Autodesk Inventor part; units mm, degrees
ref_plane "YZ Plane" through (0, 0, 0) normal (1, 0, 0) x (0, 1, 0)
ref_plane "XZ Plane" through (0, 0, 0) normal (0, 1, 0) x (-1, 0, 0)
ref_plane "XY Plane" through (0, 0, 0) normal (0, 0, 1) x (1, 0, 0)
sketch "Sketch1" plane through (0, 0, 0) normal (0, 0, 1) x (1, 0, 0)
  line L0 (0, 0) -> (-186, 0)
  line L1 (-186, 0) -> (-186, 30)
  line L2 (-186, 30) -> (0, 30)
  line L3 (0, 30) -> (0, 0)
  dimension "d0" = 186
  dimension "d1" = 30
extrude "Extrusion1" add sketch "Sketch1" along normal blind 3
sketch "Sketch2" plane through (0, 0, 0) normal (0, 0, -1) x (-1, 0, 0)
  line L0 (0, 0) -> (186, 0)
  line L1 (0, 0) -> (33, 0)
  line L2 (33, 0) -> (33, 13)
  line L3 (33, 13) -> (0, 13)
  line L4 (0, 13) -> (0, 0)
  line L5 (0, 30) -> (186, 30)
  line L6 (0, 30) -> (32.9946, 30)
  line L7 (32.9946, 30) -> (32.9946, 23)
  line L8 (32.9946, 23) -> (0, 23)
  line L9 (0, 23) -> (0, 30)
  line L10 (186, 0) -> (153, 0)
  line L11 (153, 0) -> (153, 13)
  line L12 (153, 13) -> (186, 13)
  line L13 (186, 13) -> (186, 0)
  line L14 (186, 30) -> (153, 30)
  line L15 (153, 30) -> (153, 23)
  line L16 (153, 23) -> (186, 23)
  line L17 (186, 23) -> (186, 30)
  dimension "d16" = 33
  dimension "d17" = 13
  dimension "d18" = 32.9946
  dimension "d19" = 7
  dimension "d20" = 33
hole "Hole1" at (-32.9946, 23, 0) at (-33, 13, 0) at (-153, 23, 0) at (-153, 13, 0) direction (0, 0, 1) diameter 3.4 end through all countersink diameter 6.9 countersink angle 89.954
properties part number "tyl"
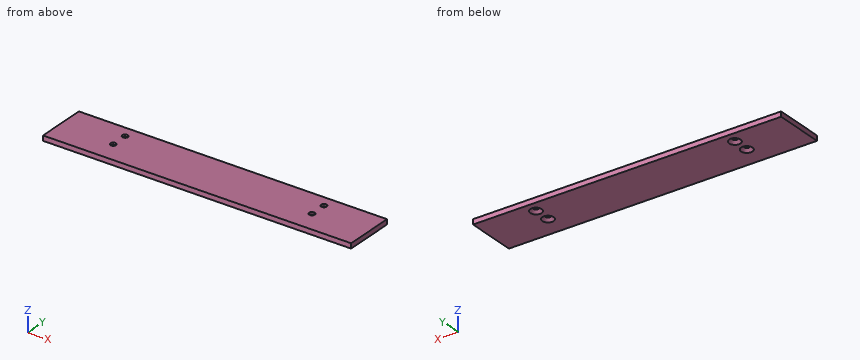
Build history of the part. All positions in model axes, mm. Coordinates: 2 decimals unless noted, no trailing zeros. Order: outer loops, then holes, each group sorted by start corner. A loop starts at its lowest first (then second) coordinate and runs counter-clockwise, first axis right, second up. Notation, with made-up numbers: (-28.5, -32) - (12.5, -32) arc R13 ccw to (12.5, -12) - close; hole circle Ø6 at (39, 7.25). An arc over 180 degrees is marked (long way). Put each result on its own line as item: value.
1. Drop flat-ended pins along their axis: P1, Ø5.5, axis at x = -33, y = 13, coming from the -Z side; P2, Ø1.5, axis at y = 5, z = 2, coming from the +X side. Give the stop position or say it passes through.
Answer sheet:
P1: stops at z = 0.7
P2: stops at x = 0
2. Probe line 1 along X through (y, z) = (23, 2.55); line 2 along Y through (x, z) = (-153, 2.45); line 3 along X through (y, z) = (21.5, 1.05). List the from-to ranges inside material, lowest first. Write a range as [from, to].
Answer sheet:
line 1: x = [-186, -154.7], [-151.3, -34.69], [-31.29, 0]
line 2: y = [0, 11.3], [14.7, 21.3], [24.7, 30]
line 3: x = [-186, -154.87], [-151.13, -34.87], [-31.12, 0]
3. Saw through at C-C (z = 0.6). Write the cut outline in (x, y), and give its area (3 significant figures).
Answer sheet:
outline: (-186, 0) - (0, 0) - (0, 30) - (-186, 30) - close; hole circle Ø5.7 at (-153, 13); hole circle Ø5.7 at (-153, 23); hole circle Ø5.7 at (-33, 13); hole circle Ø5.7 at (-32.99, 23)
area: 5,480 mm^2
4. Saw through at B-B (x = -153). Write the cut outline in (y, z), and give its area (3 significant figures).
Answer sheet:
outline: (0, 0) - (9.55, 0) - (11.3, 1.75) - (11.3, 3) - (0, 3) - close; (14.7, 1.75) - (16.45, 0) - (19.55, 0) - (21.3, 1.75) - (21.3, 3) - (14.7, 3) - close; (24.7, 1.75) - (26.45, 0) - (30, 0) - (30, 3) - (24.7, 3) - close
area: 63.5 mm^2
5. Saw through at A-A (y = 13). Write the cut outline in (x, z), and give its area (3 significant figures).
Answer sheet:
outline: (-186, 0) - (-156.45, 0) - (-154.7, 1.75) - (-154.7, 3) - (-186, 3) - close; (-151.3, 1.75) - (-149.55, 0) - (-36.45, 0) - (-34.7, 1.75) - (-34.7, 3) - (-151.3, 3) - close; (-31.3, 1.75) - (-29.55, 0) - (0, 0) - (0, 3) - (-31.3, 3) - close
area: 531 mm^2
